Autodesk Inventor part; units mm, degrees
ref_plane "YZ Plane" through (0, 0, 0) normal (1, 0, 0) x (0, 1, 0)
ref_plane "XZ Plane" through (0, 0, 0) normal (0, 1, 0) x (-1, 0, 0)
ref_plane "XY Plane" through (0, 0, 0) normal (0, 0, 1) x (1, 0, 0)
sketch "スケッチ1" plane through (0, 0, 0) normal (0, 0, 1) x (1, 0, 0)
  line L0 (-23.65, 15) -> (-23.65, -15)
  line L1 (-23.65, -15) -> (23.65, -15)
  line L2 (23.65, -15) -> (23.65, 15)
  line L3 (23.65, 15) -> (21.65, 15)
  line L4 (21.65, 15) -> (21.65, -13)
  line L5 (21.65, -13) -> (-21.65, -13)
  line L6 (-21.65, -13) -> (-21.65, 15)
  line L7 (-21.65, 15) -> (-23.65, 15)
  point P0 (0, 0)
  point P1 (0, -13)
  point P2 (23.65, 0)
  dimension "d0" = 2
  dimension "d1" = 2
  dimension "d2" = 43.3
  dimension "d3" = 30
extrude "押し出し1" add sketch "スケッチ1" along normal blind 23
sketch "スケッチ2" plane through (23.65, -15, 0) normal (1, 0, 0) x (0, 0, -1)
  line L0 (0, 30) -> (-23, 30)
  line L1 (0, 0) -> (-23, 0)
  line L2 (-16.55, 31.0334) -> (-16.55, 27)
  arc A0 (-16.55, 27) -> (-6.45, 27) centre (-11.5, 27) ccw
  line L3 (-6.45, 27) -> (-6.45, 31.0334)
  line L4 (-6.45, 31.0334) -> (-16.55, 31.0334)
  circle A1 centre (-20, 27) radius 1.3
  circle A2 centre (-17.5104, 20.9896) radius 1.3
  circle A3 centre (-11.5, 18.5) radius 1.3
  circle A4 centre (-5.4896, 20.9896) radius 1.3
  circle A5 centre (-3, 27) radius 1.3
  circle A6 centre (-5.4896, 33.0104) radius 1.3
  circle A7 centre (-11.5, 35.5) radius 1.3
  circle A8 centre (-17.5104, 33.0104) radius 1.3
  circle A9 centre (-16.5, 9.8) radius 1
  line L5 (-11.5, 27) -> (-11.5, 30) construction
  circle A10 centre (-6.5, 9.8) radius 1
  point P0 (0, 15)
  dimension "d6" = 27
  dimension "d7" = 8.5
  dimension "d8" = 2.6
  dimension "d9" = 5.05
  dimension "d12" = 360
  dimension "d14" = 2
  dimension "d15" = 5
  dimension "d16" = 9.8
extrude "押し出し2" cut sketch "スケッチ2" against normal blind 100 contours L3 A0 L2 L0 | L0 L2 L4 L3 | A1 | A2 | A3 | A4 | A5 | A9 | A10
chamfer "面取り1" distance 2 angle 45 4 edges at (22.65, 15, 0) (22.65, 15, 23) (-22.65, 15, 23) (-22.65, 15, 0)
sketch "スケッチ3" plane through (-23.65, -15, 0) normal (0, -1, 0) x (1, 0, 0)
  line L0 (0, 23) -> (47.3, 23)
  line L1 (0, 0) -> (0, 23)
  circle A0 centre (23.65, 11.5) radius 5.05
  circle A1 centre (23.65, 18.5) radius 1
  circle A2 centre (17.6396, 17.5104) radius 1.3
  circle A3 centre (23.65, 11.5) radius 8.5 construction
  line L2 (23.65, 11.5) -> (17.6396, 17.5104) construction
  line L3 (23.65, 11.5) -> (23.65, 18.5) construction
  circle A4 centre (16.65, 11.5) radius 1
  circle A5 centre (17.6396, 5.4896) radius 1.3
  circle A6 centre (23.65, 4.5) radius 1
  circle A7 centre (29.6604, 5.4896) radius 1.3
  circle A8 centre (30.65, 11.5) radius 1
  circle A9 centre (29.6604, 17.5104) radius 1.3
  circle A10 centre (11.65, 2.5) radius 1
  line L4 (23.65, 11.5) -> (16.65, 11.5) construction
  circle A11 centre (11.65, 20.5) radius 1
  circle A12 centre (35.65, 2.5) radius 1
  circle A13 centre (35.65, 20.5) radius 1
  point P0 (23.65, 0)
  point P1 (0, 11.5)
  point P2 (23.65, 23)
  dimension "d25" = 17
  dimension "d22" = 10.1
  dimension "d23" = 2
  dimension "d24" = 7
  dimension "d26" = 2.6
  dimension "d27" = 45
  dimension "d30" = 360
  dimension "d32" = 2
  dimension "d33" = 9
  dimension "d34" = 12
extrude "押し出し3" cut sketch "スケッチ3" against normal blind 10
equation "\"d1\" = d0"
properties part number "Servo_Arm" material "アルミニウム 5052"
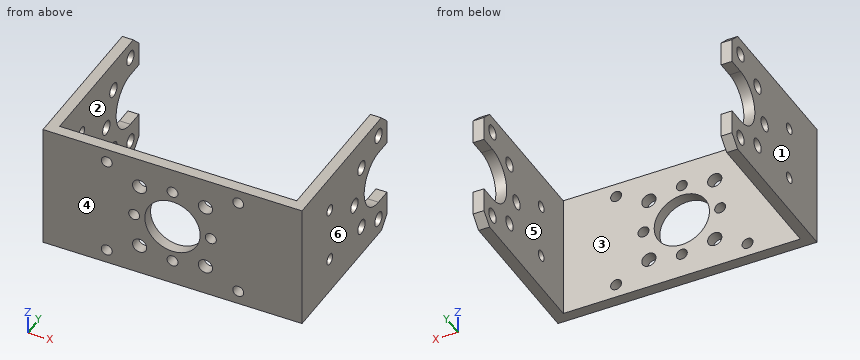
Check sheet for the modelled part. Datum: model origin and axes. Units: mm. Face numbers are marked on the shaded views. A direction names the side the tool comes from. Coordinates: 2 decimals unless noted, no trailing zeros. Loops run counter-clockwise (first coordinate to the right, second up) from the corner with the lowest first, then second, coordinate; pieces in that order, holes last. Notation, with made-up numbers: (-18, -9) -> (13, -9) arc R27 cw to (13, 9) -> close; hole circle Ø6 at (-9, 69.5). An arc over 180 degrees is marked (long way). Answer in a Markdown table with one row per item.
1. Go/stop test with flat-tipped pins: pin 1 (0.6 mm diameter, centred on x = 22.5, y = 13.5, fed in from -Z); pin 2 (11.5 mm diameter, centred on x = 0, z = 11.5, fed in from +Y). Record where each tip stops, or that it passes through.
Check values:
| item | result |
|---|---|
| pin 1 | stops at z = 0.2 |
| pin 2 | stops at y = -13 |
2. Sectioned sample at D-D, the plane z = 3. Record the boundary of the cut face in (x, y), then the cut area to 3 significant figures.
Check values:
| item | result |
|---|---|
| outline | (-23.65, -15) -> (-12.87, -15) -> (-12.87, -13) -> (-21.65, -13) -> (-21.65, 10.7) -> (-23.65, 10.7) -> close; (-23.65, 13.3) -> (-21.65, 13.3) -> (-21.65, 15) -> (-23.65, 15) -> close; (-11.13, -15) -> (11.13, -15) -> (11.13, -13) -> (-11.13, -13) -> close; (12.87, -15) -> (23.65, -15) -> (23.65, 10.7) -> (21.65, 10.7) -> (21.65, -13) -> (12.87, -13) -> close; (21.65, 13.3) -> (23.65, 13.3) -> (23.65, 15) -> (21.65, 15) -> close |
| area | 189 mm2 |
3. Sectioned sample at B-B, the plane y = -7.25. Record the boundary of the cut face in (x, z).
Check values:
| item | result |
|---|---|
| outline | (-23.65, 0) -> (-21.65, 0) -> (-21.65, 23) -> (-23.65, 23) -> close; (21.65, 0) -> (23.65, 0) -> (23.65, 23) -> (21.65, 23) -> close |
4. Access from +Z, -Z, +X, -X, +Y, -Y to the whole of each face (thin tool, end or side, straight path). Record for the marked faces 5 and 6.
Check values:
| item | result |
|---|---|
| face 5 | +Z, -Z, +Y |
| face 6 | +Z, -Z, +X, +Y, -Y |
5. Material ranges on line 1 along X through (y, z) = (-10.5, 10.5); line 2 along Y through (x, z) = (7.5, 9.5); line 3 along Y through (x, z) = (22.25, 20), recorded low to high. Write a range as [from, to].
Check values:
| item | result |
|---|---|
| line 1 | x = [-23.65, -21.65], [21.65, 23.65] |
| line 2 | y = [-15, -13] |
| line 3 | y = [-15, 10.7], [13.3, 15] |
6. Release check for a two-part mould opening along X. For the marked faces 1, 2, 3 and 4 record: released by +X, released by -X, zero draft, split by the parting line, or undercut.
Check values:
| item | result |
|---|---|
| face 1 | released by -X |
| face 2 | undercut |
| face 3 | undercut |
| face 4 | zero draft |
7. Sectioned sample at C-C, the plane x = 0. Record the boundary of the cut face in (y, z), then the cut area to 3 significant figures.
Check values:
| item | result |
|---|---|
| outline | (-15, 0) -> (-13, 0) -> (-13, 3.5) -> (-15, 3.5) -> close; (-15, 5.5) -> (-13, 5.5) -> (-13, 6.45) -> (-15, 6.45) -> close; (-15, 16.55) -> (-13, 16.55) -> (-13, 17.5) -> (-15, 17.5) -> close; (-15, 19.5) -> (-13, 19.5) -> (-13, 23) -> (-15, 23) -> close |
| area | 17.8 mm2 |
8. Sectioned sample at A-A, the plane x = -12. Record the boundary of the cut face in (y, z), then the cut area to 3 significant figures.
Check values:
| item | result |
|---|---|
| outline | (-15, 0) -> (-13, 0) -> (-13, 1.5) -> (-15, 1.5) -> close; (-15, 3.5) -> (-13, 3.5) -> (-13, 19.5) -> (-15, 19.5) -> close; (-15, 21.5) -> (-13, 21.5) -> (-13, 23) -> (-15, 23) -> close |
| area | 38.0 mm2 |
